from build123d import *

# Parameters (mm, degrees)
BOSS_EXTRUDE1_DEPTH = 1.6
BOSS_EXTRUDE2_DEPTH = 8.5
BOSS_EXTRUDE3_DEPTH = 9
SKETCH4_R           = 1.1
CUT_EXTRUDE1_DEPTH  = 2.6


with BuildPart() as part:
    # Sketch1 → Boss-Extrude1 (new body)
    with BuildSketch(Plane(origin=(0, 0, 0), x_dir=(1, 0, 0), z_dir=(0, 1, 0))):
        with BuildLine():
            Line((-10.999776277, 17.68), (-10.999776277, 33.3))
            ThreePointArc((-10.999776277, 33.3), (-8.030956433, 34.137791623), (-5, 34.711454567))
            Line((-5, 34.711454567), (-5, 24.633454567))
            Line((-5, 24.633454567), (5, 24.633454567))
            Line((5, 24.633454567), (5, 34.711454567))
            ThreePointArc((5, 34.711454567), (8.031185785, 34.137737667), (11.000223723, 33.299852195))
            Line((11.000223723, 33.299852195), (11.000223723, 17.68))
            ThreePointArc((11.000223723, 17.68), (12.956750425, 12.956526702), (17.680223723, 11))
            Line((17.680223723, 11), (33.300223723, 11))
            ThreePointArc((33.300223723, 11), (35.07, 0), (33.300223723, -11))
            Line((33.300223723, -11), (17.680223723, -11))
            ThreePointArc((17.680223723, -11), (11.24298933, -19.464492467), (21.119504048, -23.406582825))
            Line((21.119504048, -23.406582825), (30.202056601, -23.406582825))
            Line((30.202056601, -23.406582825), (36.4, -30.200102798))
            ThreePointArc((36.4, -30.200102798), (0, -47.297), (-36.4, -30.200102798))
            Line((-36.4, -30.200102798), (-30.202056601, -23.406582825))
            Line((-30.202056601, -23.406582825), (-21.119056601, -23.406582825))
            ThreePointArc((-21.119056601, -23.406582825), (-11.242541883, -19.464492467), (-17.679776277, -11))
            Line((-17.679776277, -11), (-25.999776277, -11))
            Line((-25.999776277, -11), (-25.999776277, 11))
            Line((-25.999776277, 11), (-17.679776277, 11))
            ThreePointArc((-17.679776277, 11), (-12.956302978, 12.956526702), (-10.999776277, 17.68))
        make_face()
    extrude(amount=BOSS_EXTRUDE1_DEPTH)

    # Sketch2 → Boss-Extrude2 (add)
    with BuildSketch(Plane(origin=(0, 1.6, 0), x_dir=(1, 0, 0), z_dir=(0, 1, 0))):
        Polygon((-33.597062742, -27.864051564), (-23.868298315, -36.027454207), (-20.602937258, -32.135948436), (-30.331701685, -23.972545793), align=None)
        Polygon((23.868298315, -36.027454207), (33.597062742, -27.864051564), (30.331701685, -23.972545793), (20.602937258, -32.135948436), align=None)
    extrude(amount=BOSS_EXTRUDE2_DEPTH)

    # Sketch3 → Boss-Extrude3 (add)
    with BuildSketch(Plane(origin=(0, 1.6, 0), x_dir=(1, 0, 0), z_dir=(0, 1, 0))):
        Polygon((-25.517948101, -44.939697826), (-19.990220336, -32.623276846), (-10.866945536, -36.717890005), (-16.394673301, -49.034310985), align=None)
        Polygon((-0.36916096, -38.28278004), (-2.261296496, -51.649523215), (-12.162587737, -50.247941336), (-10.2704522, -36.881198161), align=None)
        Polygon((2.261296496, -51.649523215), (0.36916096, -38.28278004), (10.2704522, -36.881198161), (12.162587737, -50.247941336), align=None)
        Polygon((16.394673301, -49.034310985), (10.866945536, -36.717890005), (19.990220336, -32.623276846), (25.517948101, -44.939697826), align=None)
    extrude(amount=BOSS_EXTRUDE3_DEPTH)

    # Sketch4 → Cut-Extrude1 (cut, through all)
    with BuildSketch(Plane(origin=(0, 1.6, 0), x_dir=(1, 0, 0), z_dir=(0, 1, 0))):
        with Locations((0, -34.8)):
            Circle(SKETCH4_R)
        with Locations((25, 0)):
            Circle(SKETCH4_R)
        with Locations((-23, 0)):
            Circle(SKETCH4_R)
        with Locations((-8, 30.5)):
            Circle(SKETCH4_R)
        with Locations((8, 30.5)):
            Circle(SKETCH4_R)
    extrude(amount=-CUT_EXTRUDE1_DEPTH, mode=Mode.SUBTRACT)


solid = part.part
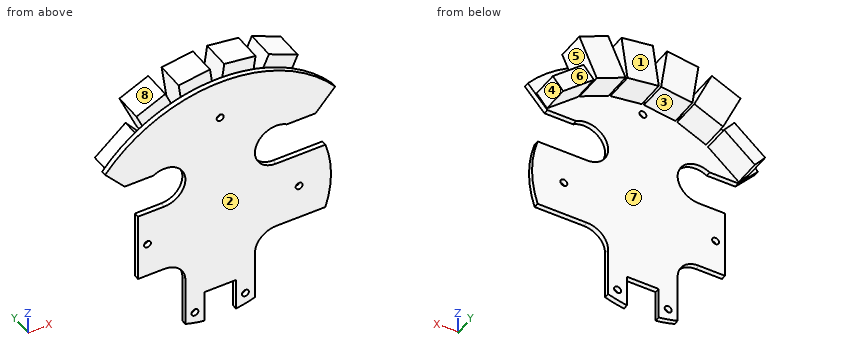
Source: CAD feature listing. Evaluate the final solid. Frame: model axes, mm. Face numbers are marked on the shaded views. A direction names the side the tool comes from. Give positions to 0.01 mm unless a question says otherwise; leave off trailing zeros. Order: outer loops, then holes, each group sorted by start corner. A loop starts at its lowest first (then second) coordinate and runs counter-clockwise, first axis right, second up. Notation, with made-up numbers: (63, -2.5) -> (112, -2.5) arc R19 cw to (112, 23.5) -> close; hole circle Ø1 at (24.5, 61.5). An arc over 180 degrees is marked (long way). Write item = value, one per line.
Item 1: Section query B-B (z = -27.5). Output: boundary loops of the cut face in (x, y).
Check result:
outline = (-11, 0) -> (-5, 0) -> (-5, 1.6) -> (-11, 1.6) -> close; (5, 0) -> (11, 0) -> (11, 1.6) -> (5, 1.6) -> close
Item 2: Section query C-C (x = 8). Output: boundary loops of the cut face in (y, z).
Check result:
outline = (0, -34.15) -> (1.6, -34.15) -> (1.6, -31.6) -> (0, -31.6) -> close; (0, -29.4) -> (1.6, -29.4) -> (1.6, 37.2) -> (10.6, 37.2) -> (10.6, 50.84) -> (1.6, 50.84) -> (1.6, 46.62) -> (0, 46.62) -> close
Item 3: Set-up query: the marked faces 1, 2, 3, 4 and 5. Return all of +Z, -Z, +X, -X, +Y, -Y with unobstructed straight access to the full face (end or side cutting, diameter ignored); none if empty.
Check result:
face_1 = +Z, -Z, +X, -X, +Y
face_2 = +Z, -Z, +X, -X, -Y
face_3 = -Z, +Y
face_4 = -Z, +X, +Y
face_5 = +Y
Item 4: Ray query, probe 1 along Z at (x, y) = (0, 0.75); probe 2 along Y at (x, z) = (15, -3); probe 3 along X at (y, z) = (0.7, 17.68). Return the intervals inside material, ascending.
Check result:
probe_1 = -24.63 to 33.7, 35.9 to 47.3
probe_2 = 0 to 1.6
probe_3 = -11 to 11
Item 5: Section query D-D (z = 0). Output: boundary loops of the cut face in (x, y).
Check result:
outline = (-26, 0) -> (-24.1, 0) -> (-24.1, 1.6) -> (-26, 1.6) -> close; (-21.9, 0) -> (23.9, 0) -> (23.9, 1.6) -> (-21.9, 1.6) -> close; (26.1, 0) -> (35.07, 0) -> (35.07, 1.6) -> (26.1, 1.6) -> close
Item 6: Section query A-A (y = 6.25). Output: boundary loops of the cut face in (x, z), then the cut area to 3 significant figures.
Check result:
outline = (-33.6, 27.86) -> (-30.33, 23.97) -> (-20.6, 32.14) -> (-23.87, 36.03) -> close; (-25.52, 44.94) -> (-19.99, 32.62) -> (-10.87, 36.72) -> (-16.39, 49.03) -> close; (-12.16, 50.25) -> (-10.27, 36.88) -> (-0.37, 38.28) -> (-2.26, 51.65) -> close; (0.37, 38.28) -> (10.27, 36.88) -> (12.16, 50.25) -> (2.26, 51.65) -> close; (10.87, 36.72) -> (19.99, 32.62) -> (25.52, 44.94) -> (16.39, 49.03) -> close; (20.6, 32.14) -> (30.33, 23.97) -> (33.6, 27.86) -> (23.87, 36.03) -> close
area = 669 mm²
Item 7: Mould query, pull axis X, two halves, no side actions, for the marked faces 6, 7 and 8. Classes: +X half, -X half, draft (parallel to the pull), parting line (faces both ways), or undercut.
Check result:
face_6 = draft
face_7 = undercut
face_8 = -X half
Item 8: Contact query for flat-ended pins moving along their axis: pin 1 (1.8 mm diameter, centred on x = 23.5, y = 0.5, fed in from -Z); pin 2 (1.8 mm diameter, centred on x = -1.5, y = 1, fed in from -Z); pin 3 (1.8 mm diameter, centred on y = 0.5, z = -26.5, fed in from +X); pin 4 (3 mm diameter, centred on x = 18.5, z = 34.5, fed in from -Y). Output: stop coordinate, or through.
Check result:
pin_1 = -11
pin_2 = -24.63
pin_3 = 11
pin_4 = 0
